from build123d import *

# Parameters (mm, degrees)
SKETCH1_W           = 110
SKETCH1_H           = 60
BOSS_EXTRUDE1_DEPTH = 50
SKETCH2_W           = 100
SKETCH2_H           = 60
CUT_EXTRUDE1_DEPTH  = 45
FILLET1_R           = 5
FILLET2_R           = 10
SKETCH3_R           = 30
CUT_EXTRUDE2_DEPTH  = 6
CUT_EXTRUDE3_DEPTH  = 6
CUT_EXTRUDE4_REACH  = 112
CUT_EXTRUDE5_REACH  = 112
SKETCH6_R           = 3
BOSS_EXTRUDE2_DEPTH = 5
CUT_EXTRUDE6_REACH  = 112
CUT_EXTRUDE9_REACH  = 112
SKETCH10_R          = 10
SKETCH10_R_2        = 3
CHAMFER1_SIZE       = 5


with BuildPart() as part:
    # Sketch1 → Boss-Extrude1 (new body)
    with BuildSketch(Plane.XY):
        with Locations((55, -30)):
            Rectangle(SKETCH1_W, SKETCH1_H)
    extrude(amount=BOSS_EXTRUDE1_DEPTH)

    # Sketch2 → Cut-Extrude1 (cut)
    with BuildSketch(Plane.XY.offset(50)):
        with Locations((55, -30)):
            Rectangle(SKETCH2_W, SKETCH2_H)
    extrude(amount=-CUT_EXTRUDE1_DEPTH, mode=Mode.SUBTRACT)

    # Fillet1
    fillet1_edges = [part.edges().sort_by_distance(p)[0] for p in [
        (5, -30, 5),
        (105, -30, 5),
    ]]
    fillet(fillet1_edges, radius=FILLET1_R)

    # Fillet2
    fillet2_edges = [part.edges().sort_by_distance(p)[0] for p in [
        (110, -30, 0),
        (0, -30, 0),
    ]]
    fillet(fillet2_edges, radius=FILLET2_R)

    # Sketch3 → Cut-Extrude2 (cut, through all)
    with BuildSketch(Plane.XY.offset(5)):
        with Locations((55, 22)):
            Circle(SKETCH3_R)
    extrude(amount=-CUT_EXTRUDE2_DEPTH, mode=Mode.SUBTRACT)

    # Sketch4 → Cut-Extrude3 (cut, through all)
    with BuildSketch(Plane.XY.offset(5)):
        with BuildLine():
            Line((20, -24), (35, -24))
            ThreePointArc((35, -24), (41, -30), (35, -36))
            Line((35, -36), (20, -36))
            ThreePointArc((20, -36), (14, -30), (20, -24))
        make_face()
        with BuildLine():
            Line((90, -24), (75, -24))
            ThreePointArc((75, -24), (69, -30), (75, -36))
            Line((75, -36), (90, -36))
            ThreePointArc((90, -36), (96, -30), (90, -24))
        make_face()
    extrude(amount=-CUT_EXTRUDE3_DEPTH, mode=Mode.SUBTRACT)

    # Sketch5 → Cut-Extrude4 (cut, up to next)
    with BuildSketch(Plane.ZY, mode=Mode.PRIVATE) as cut_extrude4_sk1:
        with BuildLine():
            Line((60, -30), (20, -30))
            ThreePointArc((20, -30), (14, -24), (20, -18))
            Line((20, -18), (60, -18))
            ThreePointArc((60, -18), (66, -24), (60, -30))
        make_face()
    cut_extrude4_tool1 = extrude(cut_extrude4_sk1.sketch, amount=-CUT_EXTRUDE4_REACH, mode=Mode.PRIVATE) & part.part
    add(cut_extrude4_tool1.solids().sort_by_distance((0, -24, 40))[0], mode=Mode.SUBTRACT)

    # Sketch6 → Cut-Extrude5 (cut, up to next)
    with BuildSketch(Plane.ZY, mode=Mode.PRIVATE) as cut_extrude5_sk1:
        with Locations((20, -10)):
            Circle(SKETCH6_R)
    cut_extrude5_tool1 = extrude(cut_extrude5_sk1.sketch, amount=-CUT_EXTRUDE5_REACH, mode=Mode.PRIVATE) & part.part
    add(cut_extrude5_tool1.solids().sort_by_distance((0, -10, 20))[0], mode=Mode.SUBTRACT)
    # Sketch6 → Cut-Extrude5 (cut, up to next)
    with BuildSketch(Plane.ZY, mode=Mode.PRIVATE) as cut_extrude5_sk2:
        with Locations((40, -10)):
            Circle(SKETCH6_R)
    cut_extrude5_tool2 = extrude(cut_extrude5_sk2.sketch, amount=-CUT_EXTRUDE5_REACH, mode=Mode.PRIVATE) & part.part
    add(cut_extrude5_tool2.solids().sort_by_distance((0, -10, 40))[0], mode=Mode.SUBTRACT)
    # Sketch6 → Cut-Extrude5 (cut, up to next)
    with BuildSketch(Plane.ZY, mode=Mode.PRIVATE) as cut_extrude5_sk3:
        with Locations((40, -50)):
            Circle(SKETCH6_R)
    cut_extrude5_tool3 = extrude(cut_extrude5_sk3.sketch, amount=-CUT_EXTRUDE5_REACH, mode=Mode.PRIVATE) & part.part
    add(cut_extrude5_tool3.solids().sort_by_distance((0, -50, 40))[0], mode=Mode.SUBTRACT)
    # Sketch6 → Cut-Extrude5 (cut, up to next)
    with BuildSketch(Plane.ZY, mode=Mode.PRIVATE) as cut_extrude5_sk4:
        with Locations((20, -50)):
            Circle(SKETCH6_R)
    cut_extrude5_tool4 = extrude(cut_extrude5_sk4.sketch, amount=-CUT_EXTRUDE5_REACH, mode=Mode.PRIVATE) & part.part
    add(cut_extrude5_tool4.solids().sort_by_distance((0, -50, 20))[0], mode=Mode.SUBTRACT)

    # Sketch8 → Boss-Extrude2 (add)
    with BuildSketch(Plane(origin=(110, 0, 0), x_dir=(0, 0, -1), z_dir=(1, 0, 0))):
        with BuildLine():
            Line((-10, -7.639320225), (-10, -52.360679775))
            ThreePointArc((-10, -52.360679775), (-60, -30), (-10, -7.639320225))
        make_face()
    extrude(amount=-BOSS_EXTRUDE2_DEPTH)

    # Sketch9 → Cut-Extrude6 (cut, up to next)
    with BuildSketch(Plane(origin=(110, 0, 0), x_dir=(0, 0, -1), z_dir=(1, 0, 0)), mode=Mode.PRIVATE) as cut_extrude6_sk1:
        with BuildLine():
            Line((-50, -7.639320225), (-50, 0))
            Line((-50, 0), (-30, 0))
            ThreePointArc((-30, 0), (-40.704662693, -1.974829231), (-50, -7.639320225))
        make_face()
    cut_extrude6_tool1 = extrude(cut_extrude6_sk1.sketch, amount=-CUT_EXTRUDE6_REACH, mode=Mode.PRIVATE) & part.part
    add(cut_extrude6_tool1.solids().sort_by_distance((110, -2.231338, 45.13628))[0], mode=Mode.SUBTRACT)
    # Sketch9 → Cut-Extrude6 (cut, up to next)
    with BuildSketch(Plane(origin=(110, 0, 0), x_dir=(0, 0, -1), z_dir=(1, 0, 0)), mode=Mode.PRIVATE) as cut_extrude6_sk2:
        with BuildLine():
            Line((-50, -60), (-30, -60))
            ThreePointArc((-30, -60), (-40.704662693, -58.025170769), (-50, -52.360679775))
            Line((-50, -52.360679775), (-50, -60))
        make_face()
    cut_extrude6_tool2 = extrude(cut_extrude6_sk2.sketch, amount=-CUT_EXTRUDE6_REACH, mode=Mode.PRIVATE) & part.part
    add(cut_extrude6_tool2.solids().sort_by_distance((110, -57.768662, 45.13628))[0], mode=Mode.SUBTRACT)

    # Sketch10 → Cut-Extrude9 (cut, up to next)
    with BuildSketch(Plane(origin=(110, 0, 0), x_dir=(0, 0, -1), z_dir=(1, 0, 0)), mode=Mode.PRIVATE) as cut_extrude9_sk1:
        with Locations((-30, -30)):
            Circle(SKETCH10_R)
    cut_extrude9_tool1 = extrude(cut_extrude9_sk1.sketch, amount=-CUT_EXTRUDE9_REACH, mode=Mode.PRIVATE) & part.part
    add(cut_extrude9_tool1.solids().sort_by_distance((110, -30, 30))[0], mode=Mode.SUBTRACT)
    # Sketch10 → Cut-Extrude9 (cut, up to next)
    with BuildSketch(Plane(origin=(110, 0, 0), x_dir=(0, 0, -1), z_dir=(1, 0, 0)), mode=Mode.PRIVATE) as cut_extrude9_sk2:
        with Locations((-44.142135624, -15.857864376)):
            Circle(SKETCH10_R_2)
    cut_extrude9_tool2 = extrude(cut_extrude9_sk2.sketch, amount=-CUT_EXTRUDE9_REACH, mode=Mode.PRIVATE) & part.part
    add(cut_extrude9_tool2.solids().sort_by_distance((110, -15.857864, 44.142136))[0], mode=Mode.SUBTRACT)
    # Sketch10 → Cut-Extrude9 (cut, up to next)
    with BuildSketch(Plane(origin=(110, 0, 0), x_dir=(0, 0, -1), z_dir=(1, 0, 0)), mode=Mode.PRIVATE) as cut_extrude9_sk3:
        with Locations((-15.857864376, -15.857864376)):
            Circle(SKETCH10_R_2)
    cut_extrude9_tool3 = extrude(cut_extrude9_sk3.sketch, amount=-CUT_EXTRUDE9_REACH, mode=Mode.PRIVATE) & part.part
    add(cut_extrude9_tool3.solids().sort_by_distance((110, -15.857864, 15.857864))[0], mode=Mode.SUBTRACT)
    # Sketch10 → Cut-Extrude9 (cut, up to next)
    with BuildSketch(Plane(origin=(110, 0, 0), x_dir=(0, 0, -1), z_dir=(1, 0, 0)), mode=Mode.PRIVATE) as cut_extrude9_sk4:
        with Locations((-15.857864376, -44.142135624)):
            Circle(SKETCH10_R_2)
    cut_extrude9_tool4 = extrude(cut_extrude9_sk4.sketch, amount=-CUT_EXTRUDE9_REACH, mode=Mode.PRIVATE) & part.part
    add(cut_extrude9_tool4.solids().sort_by_distance((110, -44.142136, 15.857864))[0], mode=Mode.SUBTRACT)
    # Sketch10 → Cut-Extrude9 (cut, up to next)
    with BuildSketch(Plane(origin=(110, 0, 0), x_dir=(0, 0, -1), z_dir=(1, 0, 0)), mode=Mode.PRIVATE) as cut_extrude9_sk5:
        with Locations((-44.142135624, -44.142135624)):
            Circle(SKETCH10_R_2)
    cut_extrude9_tool5 = extrude(cut_extrude9_sk5.sketch, amount=-CUT_EXTRUDE9_REACH, mode=Mode.PRIVATE) & part.part
    add(cut_extrude9_tool5.solids().sort_by_distance((110, -44.142136, 44.142136))[0], mode=Mode.SUBTRACT)

    # Chamfer1
    chamfer1_edges = [part.edges().sort_by_distance(p)[0] for p in [
        (2.5, -30, 50),
    ]]
    chamfer(chamfer1_edges, length=CHAMFER1_SIZE)


solid = part.part
Check sheet for the modelled part. Datum: model origin and axes. Units: mm. A direction names the side the tool comes from. Give positions to 0.01 mm unless a question says otherwise; leave off trailing zeros. Write each loop counter-clockwise with the first axis right and the second up, starting at its lowest first coordinate (ties: lowest second). Pieces come first, ordered by that corner, then holes. Notation, with made-up numbers: (3, -11.75) -> (25, -11.75) arc R27 cw to (25, 23.25) -> close; hole circle Ø10 at (10, 30). An arc over 180 degrees is marked (long way). One line per item, written item: value. Start each with the question number.
Item 1: Gauge pin test, flat ends, axial feed: pin 1 (4 mm diameter, centred on x = 72, y = -16, fed in from -Z); pin 2 (5 mm diameter, centred on y = -44.14, z = 15.86, fed in from +X); pin 3 (1 mm diameter, centred on x = 44, y = -48.5, fed in from +Z); pin 4 (4 mm diameter, centred on x = 3.5, y = -9.5, fed in from +Z). Record the tip position at first contact, or that the pin passes through.
Item 2: Section check C-C on y = -50. Record the cut outline in (x, z), then the cut area to 3 significant figures.
Item 3: Tool access check on faces 1 (the cylindrical face through (107.54, -14.96, 41.28)), 2 (the cylindrical face through (104, -30, 7)), 3 (the flat face through (82, -36, 3)). Record the directions out of +Z, -Z, +X, -X, +Y, -Y that give a thin tool (end or side, any length) a straight path to the whole face; none if there is none.
Item 4: Section check D-D on x = 52. Record the cut outline in (y, z), then the cut area to 3 significant figures.
Item 5: Draft check along Z on faces 4 (the cylindrical face through (2, -47, 20)), 5 (the flat face through (98, 0, 4)), 6 (the cylindrical face through (7, -30, 6)). Enter one of: +Z half, -Z half, draft (parallel to the pull), parting line (faces both ways), or undercut.
Item 6: Section check B-B on y = -25.5. Record the cut outline in (x, z), then the cut area to 3 significant figures.
Item 7: Material ranges on probe 1 along X at (y, z) = (-44, 25); probe 2 along X at (y, z) = (-30, 3.5); probe 3 along X at (y, z) = (-20, 45), recorded low to high. Write a range as from..to.
Item 8: Section check A-A on x = 26.5. Record the cut outline in (y, z).
Results list:
1. pin 1: z = 0
1. pin 2: x = 5
1. pin 3: z = 5
1. pin 4: z = 50
2. outline: (0, 10) arc R10 ccw to (10, 0) -> (100, 0) arc R10 ccw to (110, 10) -> (110, 52.36) -> (105, 52.36) -> (105, 10) arc R5 cw to (100, 5) -> (10, 5) arc R5 cw to (5, 10) -> (5, 17) -> (0, 17) -> close; (0, 23) -> (5, 23) -> (5, 37) -> (0, 37) -> close; (0, 43) -> (5, 43) -> (5, 50) -> (0, 50) -> close
2. area: 920 mm²
3. face 1: +X
3. face 2: +Z, +Y, -Y
3. face 3: +Z, -Z
4. outline: (-60, 0) -> (-7.85, 0) -> (-7.85, 5) -> (-60, 5) -> close
4. area: 261 mm²
5. face 4: undercut
5. face 5: draft
5. face 6: +Z half
6. outline: (0, 10) arc R10 ccw to (10, 0) -> (16.03, 0) -> (16.03, 5) -> (10, 5) arc R5 cw to (5, 10) -> (5, 14.19) -> (0, 14.19) -> close; (38.97, 0) -> (71.03, 0) -> (71.03, 5) -> (38.97, 5) -> close; (93.97, 0) -> (100, 0) arc R10 ccw to (110, 10) -> (110, 21.07) -> (105, 21.07) -> (105, 10) arc R5 cw to (100, 5) -> (93.97, 5) -> close; (105, 38.93) -> (110, 38.93) -> (110, 59.66) -> (105, 59.66) -> close
6. area: 518 mm²
7. probe 1: 0..5, 105..110
7. probe 2: 2.4..14, 41..69, 96..107.6
7. probe 3: 105..110
8. outline: (-60, 0) -> (-36, 0) -> (-36, 5) -> (-60, 5) -> close; (-24, 0) -> (0, 0) -> (0, 5) -> (-24, 5) -> close
